Work out the finished part from the listing and answer in its coordinate system (mm). A direction names the side the tool comes from. Give positions to 0.01 mm unless a question says otherwise; leave off trailing zeros. Write each loop counter-clockwise with the first axis right and the second up, starting at its lowest first coordinate (ties: lowest second). Pieces come first, ordered by that corner, then holes.
1) Find section A-A (z = 7.5). Determine the outline of the cut face in (x, y), plus the area to 3 significant figures.
2) A tool of negligible diameter and unlimited length cuts with its end or side. For faces 4 (the face through (-24, 24, 0)), 5 (the face through (-27.21, 22.48, 5.47)), from which of +Z, -Z, +X, -X, +Y, -Y can it reach the whole face along a straight path? Write none if from no direction.
3) Find section D-D (x = -29.25). Determine the outline of the cut face in (y, z), plus the area to 3 significant figures.
4) Find section B-B (y = 37). Determine the outline of the cut face in (x, z).
5) Determine the mould class of faces 1 (the face through (-12.48, 39.53, -9.11)), 2 (the face through (-14, 38, 0)), 3 (the face through (-13, 31, -15)) for opening direction Z: pulls with the +Z half, pulls with the -Z half, needs draft (parallel to the pull), parting line crosses it, or undercut.
6) Find section C-C (z = -8.75). Determine the outline of the cut face in (x, y).
7) Given pin 1 Ø4 at (x, z) = (-32, 9.5) entering from +Y; pin 2 Ø3.5 at (x, z) = (-25, -7.5) entering from +Y; pin 3 Ø8 at (x, y) = (-18, 27) entering from -Z; pin 4 Ø1 at (y, z) = (28, -1) entering from -X, each flat-ended and moving along its own axis, determine where each tip first touches the part or whether it passes through.
8) Straight lines are drawn through the part: probe 1 along Z at (x, y) = (-25, 23.25); probe 2 along X at (y, z) = (22.85, -7.5); probe 3 along Y at (x, z) = (-13.3, 7.5). For each, find the intervals that lie inside material, in ascending order.
```python
from build123d import *

# Parameters (mm, degrees)
AUFSATZ_LINEAR_AUSTRAGEN1_DEPTH      = 15
AUFSATZ_LINEAR_AUSTRAGEN1_DEPTH_BACK = 15
SKIZZE6_R                            = 3
SCHNITT_LINEAR_AUSTRAGEN1_DEPTH      = 14
SKIZZE8_R                            = 3
SCHNITT_LINEAR_AUSTRAGEN2_DEPTH      = 24


with BuildPart() as part:
    # Skizze3 → Aufsatz-Linear austragen1 (new body, two sides)
    with BuildSketch(Plane.XY) as aufsatz_linear_austragen1_sk:
        Polygon((-14, 24), (-35, 24), (-35, 21), (-11, 21), (-11, 51), (-14, 51), align=None)
    extrude(amount=AUFSATZ_LINEAR_AUSTRAGEN1_DEPTH)
    extrude(aufsatz_linear_austragen1_sk.sketch, amount=-AUFSATZ_LINEAR_AUSTRAGEN1_DEPTH_BACK)

    # Skizze6 → Schnitt-Linear austragen1 (cut)
    with BuildSketch(Plane(origin=(0, 0, 0), x_dir=(0, 0, -1), z_dir=(1, 0, 0))):
        with Locations((7.5, 37)):
            Circle(SKIZZE6_R)
        with Locations((-7.5, 37)):
            Circle(SKIZZE6_R)
    extrude(amount=-SCHNITT_LINEAR_AUSTRAGEN1_DEPTH, mode=Mode.SUBTRACT)

    # Skizze8 → Schnitt-Linear austragen2 (cut)
    with BuildSketch(Plane(origin=(0, 0, 0), x_dir=(1, 0, 0), z_dir=(0, 1, 0))):
        with Locations((-25, 7.5)):
            Circle(SKIZZE8_R)
        with Locations((-25, -7.5)):
            Circle(SKIZZE8_R)
    extrude(amount=SCHNITT_LINEAR_AUSTRAGEN2_DEPTH, mode=Mode.SUBTRACT)


solid = part.part
```
Results:
1. outline: (-35, 21) - (-28, 21) - (-28, 24) - (-35, 24) - close; (-22, 21) - (-11, 21) - (-11, 34) - (-14, 34) - (-14, 24) - (-22, 24) - close; (-14, 40) - (-11, 40) - (-11, 51) - (-14, 51) - close
1. area: 117 mm2
2. face 4: +Z, -Z, -X, +Y
2. face 5: +Y, -Y
3. outline: (21, -15) - (24, -15) - (24, 15) - (21, 15) - close
3. area: 90.0 mm2
4. outline: (-14, -15) - (-11, -15) - (-11, -10.5) - (-14, -10.5) - close; (-14, -4.5) - (-11, -4.5) - (-11, 4.5) - (-14, 4.5) - close; (-14, 10.5) - (-11, 10.5) - (-11, 15) - (-14, 15) - close
5. face 1: undercut
5. face 2: needs draft
5. face 3: pulls with the -Z half
6. outline: (-35, 21) - (-27.73, 21) - (-27.73, 24) - (-35, 24) - close; (-22.27, 21) - (-11, 21) - (-11, 34.27) - (-14, 34.27) - (-14, 24) - (-22.27, 24) - close; (-14, 39.73) - (-11, 39.73) - (-11, 51) - (-14, 51) - close
7. pin 1: stops at y = 24
7. pin 2: passes through
7. pin 3: stops at z = -15
7. pin 4: stops at x = -14
8. probe 1: z = -15 to -10.5, -4.5 to 4.5, 10.5 to 15
8. probe 2: x = -35 to -28, -22 to -11
8. probe 3: y = 21 to 34, 40 to 51
